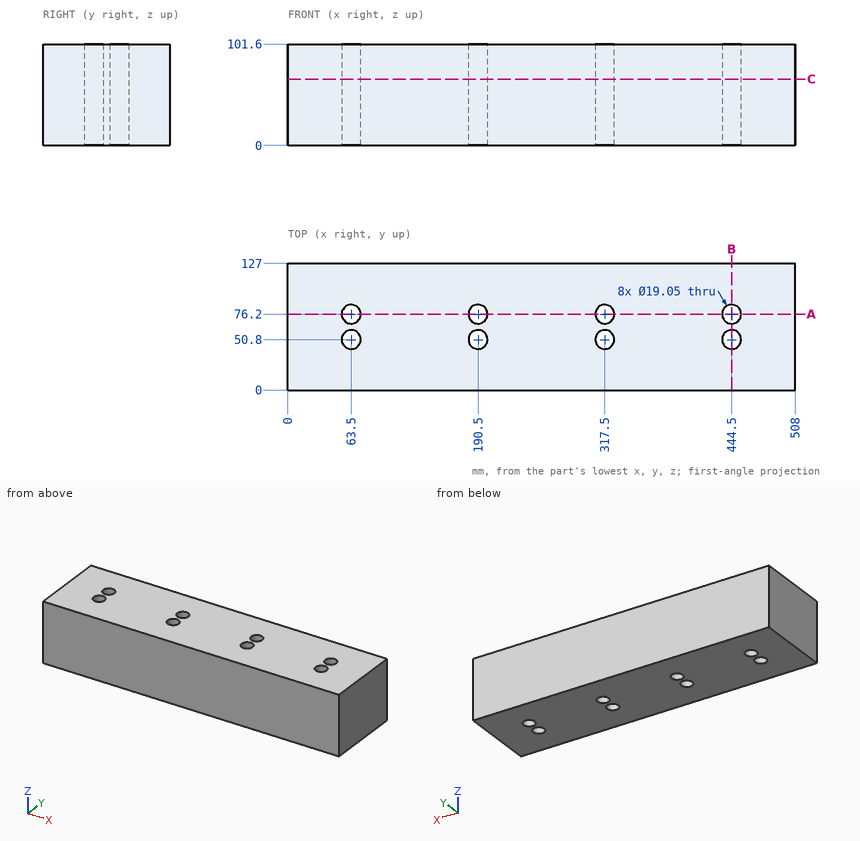
Source: three-view drawing plus pictorial views. Frame: mm from the lowest corner of the part. Round coordinates to 2 decimals unless told otherwise and drop trailing zeros. Loops run counter-clockwise (first coordinate to the right, second up) from the corner with the lowest first, then second, coordinate; pieces in that order, holes last. Notation, with made-up numbers: (67.25, 74.5) - (79.25, 74.5) arc R16 ccw to (79.25, 98.5) - close; hole circle Ø6 at (9, -9). An arc over 180 degrees is marked (long way). Write each question's results on one line, items separated by ' | '. Start each with the question number.
1) Cut plane A-A on y = 76.2. Return loops of the section in (x, z) (3 decimals).
2) Cut plane C-C on z = 66.5. Count the separate pieces of the cut face and the enclosed holes in it, then the cut area to 3 significant figures.
3) Line query: probe 1 along Y at (x, z) = (190.5, 33.5) (3 decimals); probe 2 along X at (y, z) = (84, 93); probe 3 along X at (y, z) = (72.5, 85). Output: solid intervals per line, ascending. Write a range as [from, to].
4) Cut plane B-B on x = 444.5. Return loops of the section in (y, z) (3 decimals), then the cut area to 3 significant figures.
Verdict:
1) outline: (0, 0) - (53.975, 0) - (53.975, 101.6) - (0, 101.6) - close; (73.025, 0) - (180.975, 0) - (180.975, 101.6) - (73.025, 101.6) - close; (200.025, 0) - (307.975, 0) - (307.975, 101.6) - (200.025, 101.6) - close; (327.025, 0) - (434.975, 0) - (434.975, 101.6) - (327.025, 101.6) - close; (454.025, 0) - (508, 0) - (508, 101.6) - (454.025, 101.6) - close
2) separate pieces: 1 | enclosed holes: 8 | area: 62,200 mm2
3) probe 1: y = [0, 41.275], [60.325, 66.675], [85.725, 127] | probe 2: x = [0, 58.03], [68.97, 185.03], [195.97, 312.03], [322.97, 439.03], [449.97, 508] | probe 3: x = [0, 54.72], [72.28, 181.72], [199.28, 308.72], [326.28, 435.72], [453.28, 508]
4) outline: (0, 0) - (41.275, 0) - (41.275, 101.6) - (0, 101.6) - close; (60.325, 0) - (66.675, 0) - (66.675, 101.6) - (60.325, 101.6) - close; (85.725, 0) - (127, 0) - (127, 101.6) - (85.725, 101.6) - close | area: 9,030 mm2
